Source: CAD feature listing. Evaluate the final solid. Frame: model axes, mm. A direction names the side the tool comes from. Coordinates: 2 decimals unless noted, no trailing zeros. Write each loop counter-clockwise with the first axis right and the second up, starting at its lowest first coordinate (ties: lowest second). Pieces come first, ordered by that corner, then holes. Notation, with made-up numbers: (55.25, 18.5) -> (104.25, 18.5) arc R19 ccw to (104.25, 53.5) -> close; hole circle Ø2 at (73.25, -29). An arc over 180 degrees is marked (long way). One line per item, written item: value. Start each with the question number.
1. Access query for faces 5 (the flat face through (-40, 4, -1)), 6 (the cylindrical face through (-21.96, 23.22, -1.32)), 7 (the flat face through (33.8, -1, -1)). Directions: +Z, -Z, +X, -X, +Y, -Y. A direction counts if a zero-diameter tool reaches every point of the face in a straight line with its end or side. Return the directions, or none.
2. Section query B-B, the plane x = 36.4. Output: boundary loops of the cut face in (y, z).
3. Section query A-A, the plane y = 28.65. Output: boundary loops of the cut face in (x, z).
4. Mould query, pull axis X, two halves, no side actions, for faces 1 (the cylindrical face through (-32.316, -25.778, -1.318)), 2 (the cylindrical face through (39.218, -31.759, -1.318)), 3 (the cylindrical face through (-21.98, 14.16, -1.32)), 4 (the cylindrical face through (-9.078, 22.484, -1.318)). Classes: released by +X, released by -X, zero draft, split by the parting line, or undercut.
5. Section query C-C, the plane x = -36.4. Output: boundary loops of the cut face in (y, z), and give its area (3 significant figures).
6. Section query D-D, the plane y = -23. Output: boundary loops of the cut face in (x, z), and give its area (3 significant figures).
7. Line query: line 1 (Y direction, x = 1.5, z = -0.1); line 2 (Y direction, x = 36.4, z = -0.85); line 3 (Y direction, x = -36.4, z = -1.7). Output: solid intervals per line, ascending.
from build123d import *

# Parameters (mm, degrees)
SKETCH1_W          = 80
SKETCH1_H          = 65
BASE_FLANGE1_DEPTH = 2.6
SKETCH6_R          = 1.0999978
CUT_EXTRUDE1_DEPTH = 10
FILLET1_R          = 2.6
SKETCH7_W          = 18.5
SKETCH7_H          = 10
SKETCH7_W_2        = 43
SKETCH7_H_2        = 5
SKETCH7_W_3        = 7
CUT_EXTRUDE2_DEPTH = 2.6
FILLET2_R          = 2.4
FILLET3_R          = 1.6
SKETCH11_W         = 3.5
SKETCH11_H         = 2.8
SKETCH11_W_2       = 2.8
SKETCH11_H_2       = 3.5
CUT_EXTRUDE5_DEPTH = 10


# Sheet-metal steps are written as plain solids
with BuildPart() as part:
    # Sketch1 → Base-Flange1 (new body)
    with BuildSketch(Plane.XY):
        Rectangle(SKETCH1_W, SKETCH1_H)
    extrude(amount=-BASE_FLANGE1_DEPTH)

    # Sketch6 → Cut-Extrude1 (cut)
    with BuildSketch(Plane.XY):
        with Locations((-36.4, 28.65)):
            Circle(SKETCH6_R)
        with Locations(Location((-36.4, -28.65, 0), (0, 0, 180))):
            Circle(SKETCH6_R)
        with Locations((36.4, -28.65)):
            Circle(SKETCH6_R)
        with Locations(Location((36.4, 28.65, 0), (0, 0, 180))):
            Circle(SKETCH6_R)
    extrude(amount=-CUT_EXTRUDE1_DEPTH, mode=Mode.SUBTRACT)

    # Fillet1
    fillet1_edges = [part.edges().sort_by_distance(p)[0] for p in [
        (-40, 32.5, -1.3),
        (40, 32.5, -1.3),
        (40, -32.5, -1.3),
        (-40, -32.5, -1.3),
    ]]
    fillet(fillet1_edges, radius=FILLET1_R)

    # Sketch7 → Cut-Extrude2 (cut)
    with BuildSketch(Plane.XY):
        with Locations((-30.75, 18.7)):
            Rectangle(SKETCH7_W, SKETCH7_H)
        Polygon((-40, -4.5), (-24, -4.5), (-24, -26.5), (-33, -26.5), (-33, -17.5), (-40, -17.5), align=None)
        with Locations((11.7, 24.3)):
            Rectangle(SKETCH7_W_2, SKETCH7_H_2)
        Polygon((-11.8, -21.8), (-11.8, -16.3), (-20.8, -16.3), (-20.8, -26.8), (33.2, -26.8), (33.2, -21.8), align=None)
        with Locations((30.3, -0.8)):
            Rectangle(SKETCH7_W_3, SKETCH7_H)
    extrude(amount=-CUT_EXTRUDE2_DEPTH, mode=Mode.SUBTRACT)

    # Fillet2
    fillet2_edges = [part.edges().sort_by_distance(p)[0] for p in [
        (-9.8, 21.8, -1.3),
        (-9.8, 26.8, -1.3),
        (33.2, 26.8, -1.3),
        (33.2, 21.8, -1.3),
        (33.2, -21.8, -1.3),
        (33.2, -26.8, -1.3),
        (-20.8, -26.8, -1.3),
        (-11.8, -21.8, -1.3),
        (-24, -26.5, -1.3),
        (-33, -26.5, -1.3),
    ]]
    fillet(fillet2_edges, radius=FILLET2_R)

    # Fillet3
    fillet3_edges = [part.edges().sort_by_distance(p)[0] for p in [
        (26.8, -5.8, -1.3),
        (26.8, 4.2, -1.3),
        (33.8, 4.2, -1.3),
        (33.8, -5.8, -1.3),
        (-20.8, -16.3, -1.3),
        (-11.8, -16.3, -1.3),
        (-21.5, 23.7, -1.3),
        (-21.5, 13.7, -1.3),
        (-24, -4.5, -1.3),
    ]]
    fillet(fillet3_edges, radius=FILLET3_R)

    # Sketch11 → Cut-Extrude5 (cut)
    with BuildSketch(Plane.XY):
        with Locations((0, 28.9)):
            Rectangle(SKETCH11_W, SKETCH11_H)
        with Locations((36.55, 0)):
            Rectangle(SKETCH11_W_2, SKETCH11_H_2)
        with Locations((0, -28.9)):
            Rectangle(SKETCH11_W, SKETCH11_H)
        with Locations((-36.55, 0)):
            Rectangle(SKETCH11_W_2, SKETCH11_H_2)
    extrude(amount=-CUT_EXTRUDE5_DEPTH, mode=Mode.SUBTRACT)


solid = part.part
Computed values:
1. face 5: +Z, -Z, -X, +Y, -Y
1. face 6: +Z, -Z, -X
1. face 7: +Z, -Z
2. outline: (-32.5, -2.6) -> (-29.75, -2.6) -> (-29.75, 0) -> (-32.5, 0) -> close; (-27.55, -2.6) -> (-1.75, -2.6) -> (-1.75, 0) -> (-27.55, 0) -> close; (1.75, -2.6) -> (27.55, -2.6) -> (27.55, 0) -> (1.75, 0) -> close; (29.75, -2.6) -> (32.5, -2.6) -> (32.5, 0) -> (29.75, 0) -> close
3. outline: (-40, -2.6) -> (-37.5, -2.6) -> (-37.5, 0) -> (-40, 0) -> close; (-35.3, -2.6) -> (-1.75, -2.6) -> (-1.75, 0) -> (-35.3, 0) -> close; (1.75, -2.6) -> (35.3, -2.6) -> (35.3, 0) -> (1.75, 0) -> close; (37.5, -2.6) -> (40, -2.6) -> (40, 0) -> (37.5, 0) -> close
4. face 1: undercut
4. face 2: released by +X
4. face 3: released by -X
4. face 4: undercut
5. outline: (-32.5, -2.6) -> (-29.75, -2.6) -> (-29.75, 0) -> (-32.5, 0) -> close; (-27.55, -2.6) -> (-17.5, -2.6) -> (-17.5, 0) -> (-27.55, 0) -> close; (-4.5, -2.6) -> (-1.75, -2.6) -> (-1.75, 0) -> (-4.5, 0) -> close; (1.75, -2.6) -> (13.7, -2.6) -> (13.7, 0) -> (1.75, 0) -> close; (23.7, -2.6) -> (27.55, -2.6) -> (27.55, 0) -> (23.7, 0) -> close; (29.75, -2.6) -> (32.5, -2.6) -> (32.5, 0) -> (29.75, 0) -> close
5. area: 88.7 mm²
6. outline: (-40, -2.6) -> (-33, -2.6) -> (-33, 0) -> (-40, 0) -> close; (-24, -2.6) -> (-20.8, -2.6) -> (-20.8, 0) -> (-24, 0) -> close; (32.88, -2.6) -> (40, -2.6) -> (40, 0) -> (32.88, 0) -> close
6. area: 45.0 mm²
7. line 1: y = -32.5 to -30.3, -27.5 to -26.8, -21.8 to 21.8, 26.8 to 27.5, 30.3 to 32.5
7. line 2: y = -32.5 to -29.75, -27.55 to -1.75, 1.75 to 27.55, 29.75 to 32.5
7. line 3: y = -32.5 to -29.75, -27.55 to -17.5, -4.5 to -1.75, 1.75 to 13.7, 23.7 to 27.55, 29.75 to 32.5
